Source: CAD feature listing. Evaluate the final solid. Frame: model axes, mm. Round coordinates to 2 decimals unless told otherwise and drop trailing zeros. Order: outer loops, then holes, each group sorted by start corner. A loop starts at its lowest first (then second) coordinate and runs counter-clockwise, first axis right, second up. Notation, with made-up numbers: (45, 60) - (88, 60) arc R27 cw to (88, 94) - close; hole circle Ø8 at (37, -35.75). An arc over 180 degrees is marked (long way). Put each result on its own line as item: value. Start each with the question number.
1) Section C-C on x = 53. Output: boundary loops of the cut face in (y, z).
2) Section D-D on z = 0. State how many separate pieces and enclosed holes the cut face has, then the cut area to 3 significant figures.
3) Section B-B on y = -3.5. Output: boundary loops of the cut face in (x, z), then the cut area to 3 significant figures.
4) Line query: probe 1 along X at (y, z) = (7.1, 0); probe 2 along Y at (x, z) = (132, 1.75); probe 3 along Z at (x, y) = (140, 6.3). Output: solid intervals per line, ascending. Write a range as [from, to].
5) Section A-A on x = 140. Output: boundary loops of the cut face in (y, z).
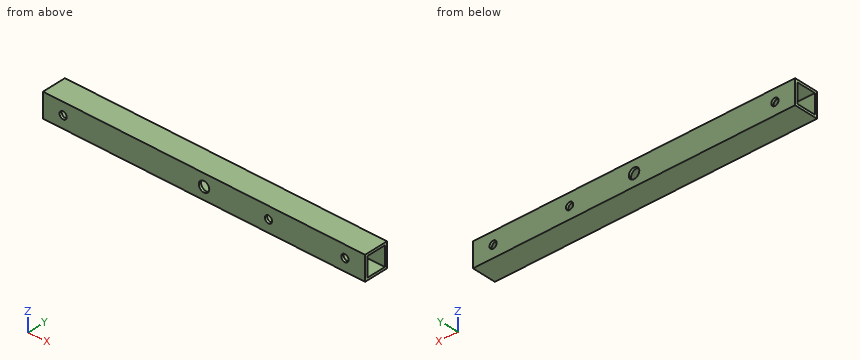
```python
from build123d import *

# Parameters (mm, degrees)
SKETCH1_W           = 15
SKETCH1_H           = 15
SKETCH1_W_2         = 12
SKETCH1_H_2         = 12
BOSS_EXTRUDE1_DEPTH = 200
SKETCH2_R           = 3.25
SKETCH2_R_2         = 2.25
CUT_EXTRUDE1_DEPTH  = 16
SKETCH3_R           = 2.25
CUT_EXTRUDE2_DEPTH  = 16


with BuildPart() as part:
    # Sketch1 → Boss-Extrude1 (new body)
    with BuildSketch(Plane(origin=(0, 0, 0), x_dir=(0, 0, -1), z_dir=(1, 0, 0))):
        Rectangle(SKETCH1_W, SKETCH1_H)
        Rectangle(SKETCH1_W_2, SKETCH1_H_2, mode=Mode.SUBTRACT)
    extrude(amount=BOSS_EXTRUDE1_DEPTH)

    # Sketch2 → Cut-Extrude1 (cut, through all)
    with BuildSketch(Plane(origin=(0, 7.5, 0), x_dir=(1, 0, 0), z_dir=(0, 1, 0))):
        with Locations((100, 0)):
            Circle(SKETCH2_R)
        with Locations((140, 0)):
            Circle(SKETCH2_R_2)
    extrude(amount=-CUT_EXTRUDE1_DEPTH, mode=Mode.SUBTRACT)

    # Sketch3 → Cut-Extrude2 (cut, through all)
    with BuildSketch(Plane(origin=(0, 7.5, 0), x_dir=(1, 0, 0), z_dir=(0, 1, 0))):
        with Locations((12.5, 0)):
            Circle(SKETCH3_R)
        with Locations((187.5, 0)):
            Circle(SKETCH3_R)
    extrude(amount=-CUT_EXTRUDE2_DEPTH, mode=Mode.SUBTRACT)


solid = part.part
```
Answer sheet:
1. outline: (-7.5, -7.5) - (7.5, -7.5) - (7.5, 7.5) - (-7.5, 7.5) - close; hole (-6, -6) - (6, -6) - (6, 6) - (-6, 6) - close
2. separate pieces: 10
2. enclosed holes: 0
2. area: 540 mm^2
3. outline: (0, -7.5) - (200, -7.5) - (200, -6) - (0, -6) - close; (0, 6) - (200, 6) - (200, 7.5) - (0, 7.5) - close
3. area: 600 mm^2
4. probe 1: [0, 10.25], [14.75, 96.75], [103.25, 137.75], [142.25, 185.25], [189.75, 200]
4. probe 2: [-7.5, -6], [6, 7.5]
4. probe 3: [-7.5, -2.25], [2.25, 7.5]
5. outline: (-7.5, -7.5) - (7.5, -7.5) - (7.5, -2.25) - (6, -2.25) - (6, -6) - (-6, -6) - (-6, -2.25) - (-7.5, -2.25) - close; (-7.5, 2.25) - (-6, 2.25) - (-6, 6) - (6, 6) - (6, 2.25) - (7.5, 2.25) - (7.5, 7.5) - (-7.5, 7.5) - close
